from build123d import *

# Parameters (mm, degrees)
PAD_DEPTH         = 270
PAD001_DEPTH      = 29
PAD002_DEPTH      = 117.5
POCKET_DEPTH      = 341.0745213347
POCKET_DEPTH_BACK = 71.6303346662


with BuildPart() as part:
    # Sketch001 → Pad (new body, symmetric)
    with BuildSketch(Plane.YZ):
        Polygon((-24.8576477137, 122.9970951405), (-9.9147272423, 121.6897589993), (12.9476758379, 58.8758227821), (22.9096228188, 58.0042653546), (5.6527857547, -139.2422848675), (-4.3091612262, -138.3707274401), (-38.1967657639, -201.5754205315), (-52.8330949144, -196.7637295572), align=None)
    extrude(amount=PAD_DEPTH, both=True)

    # Sketch002 → Pad001 (join, symmetric)
    with BuildSketch(Plane.YZ):
        with BuildLine():
            Line((62.4443669874, 107.4083042285), (85.4014673511, 106.0041878192))
            Line((85.4014673511, 106.0041878192), (62.9356048023, -261.309418))
            Line((62.9356048023, -261.309418), (39.892625, -261.309418))
            Line((39.892625, -261.309418), (52.1882123456, -60.2783419063))
            Line((34.8975714525, -60.2783419063), (52.1882123456, -60.2783419063))
            ThreePointArc((26.8824790431, -57.7511929769), (30.6955425365, -59.6315877978), (34.8975714525, -60.2783419063))
            Line((26.8824790431, -57.7511929769), (25.6252451745, -59.5467090202))
            Line((25.6252451745, -59.5467090202), (12.6252451745, -59.5467090202))
            Line((15.0656059715, -31.6532574736), (12.6252451745, -59.5467090202))
            Line((15.0656059715, -31.6532574736), (28.0656059715, -31.6532574736))
            Line((28.0656059715, -31.6532574736), (28.9919515436, -33.6398119639))
            ThreePointArc((34.8975714525, -32.3305675505), (31.8730687065, -32.6618044727), (28.9919515436, -33.6398119639))
            Line((34.8975714525, -32.3305675505), (53.8975714525, -32.3305675505))
            Line((53.8975714525, -32.3305675505), (62.4443669874, 107.4083042285))
        make_face()
    extrude(amount=PAD001_DEPTH, both=True)

    # Sketch003 → Pad002 (join, symmetric)
    with BuildSketch(Plane.YZ):
        Polygon((-92.107375, -261.309418), (101.892625, -261.309418), (101.892625, -265.309418), (95.892625, -265.309418), (95.892625, -274.309418), (-86.107375, -274.309418), (-86.107375, -265.309418), (-92.107375, -265.309418), align=None)
    extrude(amount=PAD002_DEPTH, both=True)

    # Sketch004 (on DatumPlane) → Pocket (cut, two sides)
    with BuildSketch(Plane(origin=(0, 5.210191812, 59.5527649186), x_dir=(0, -0.9961946981, 0.0871557427), z_dir=(0, 0.0871557427, 0.9961946981))) as pocket_sk:
        Polygon((20.4829600422, 270), (-7.7670399578, 209.4176794956), (-17.7670399578, 209.4176794956), (-17.7670399578, 270), align=None)
        Polygon((20.4829600422, -270), (-7.7670399578, -209.4176794956), (-17.7670399578, -209.4176794956), (-17.7670399578, -270), align=None)
    extrude(amount=-POCKET_DEPTH, mode=Mode.SUBTRACT)
    extrude(pocket_sk.sketch, amount=POCKET_DEPTH_BACK, mode=Mode.SUBTRACT)


solid = part.part
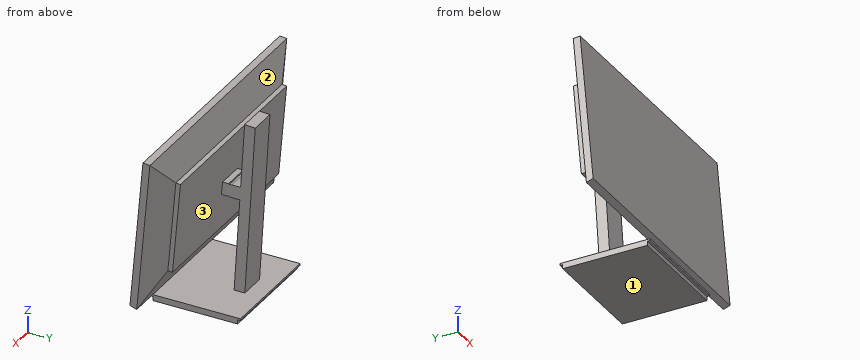
Here's how the part is built. I have some questions about the finished solid (model axes, mm). Face numbers are marked on the shaded views. Round coordinates to 2 decimals unless told otherwise and drop trailing zeros. Loops run counter-clockwise (first coordinate to the right, second up) from the corner with the lowest first, then second, coordinate; pieces in that order, holes last.
1. If we section it at A-A on x = 109: Write out the boundary of the cut face in (y, z).
Answer list:
outline: (-92.11, -265.31) - (-86.11, -265.31) - (-86.11, -274.31) - (95.89, -274.31) - (95.89, -265.31) - (101.89, -265.31) - (101.89, -261.31) - (-92.11, -261.31) - close; (-52.83, -196.76) - (-38.2, -201.58) - (-4.31, -138.37) - (5.65, -139.24) - (22.91, 58) - (12.95, 58.88) - (-9.91, 121.69) - (-24.86, 123) - close
2. If we section it at D-D on x = -184: Write out the boundary of the cut face in (y, z), plus the area to 3 significant figures.
Answer list:
outline: (-52.83, -196.76) - (-38.2, -201.58) - (-4.31, -138.37) - (5.65, -139.24) - (22.91, 58) - (12.95, 58.88) - (-9.91, 121.69) - (-24.86, 123) - close
area: 14,200 mm2
3. If we section it at B-B on z = 84: Write out the boundary of the cut face in (x, y).
Answer list:
outline: (-270, -28.27) - (270, -28.27) - (270, -13.21) - (233.65, 3.8) - (-233.65, 3.8) - (-270, -13.21) - close; (-29, 61.01) - (29, 61.01) - (29, 84.06) - (-29, 84.06) - close
4. If I drill on line 1 along X through (y, z) = (6, -81); line 2 along Y through (x, z) = (20, 2); line 3 along Z through (x, y) = (38, 49.5), over which ranges is the centre line in solid material (lowest first)?
Answer list:
line 1: x = -209.42 to 209.42
line 2: y = -35.44 to 18.01, 56 to 79.04
line 3: z = -274.31 to -261.31
5. We'd pull the mould along Z, two halves only. Please class the marked faces 1, 2 and 3: +Z half, -Z half, draft (parallel to the pull), parting line (faces both ways), or undercut.
Answer list:
face 1: -Z half
face 2: +Z half
face 3: undercut
6. If we section it at C-C on y = -44: Write out the boundary of the cut face in (x, z).
Answer list:
outline: (-270, -199.67) - (270, -199.67) - (270, -95.8) - (-270, -95.8) - close; (-117.5, -274.31) - (117.5, -274.31) - (117.5, -261.31) - (-117.5, -261.31) - close
7. For P1, Ø22, axis at y = 60.5, z = -156.5, coming from the -X side; P2, Ø4, axis at x = 206.5, z = -171.5, coming from the +Y side; P3, Ø13.5, axis at y = 7.5, z = -53.5, coming from the -X side; P4, Ø10, axis at x = 124, y = 40.5, coming from the +Z side, each with a flat end and sliding along its axis, tell me the tip position at first contact or that it passes through.
Answer list:
P1: stops at x = -29
P2: stops at y = -21
P3: stops at x = -214.53
P4: passes through
